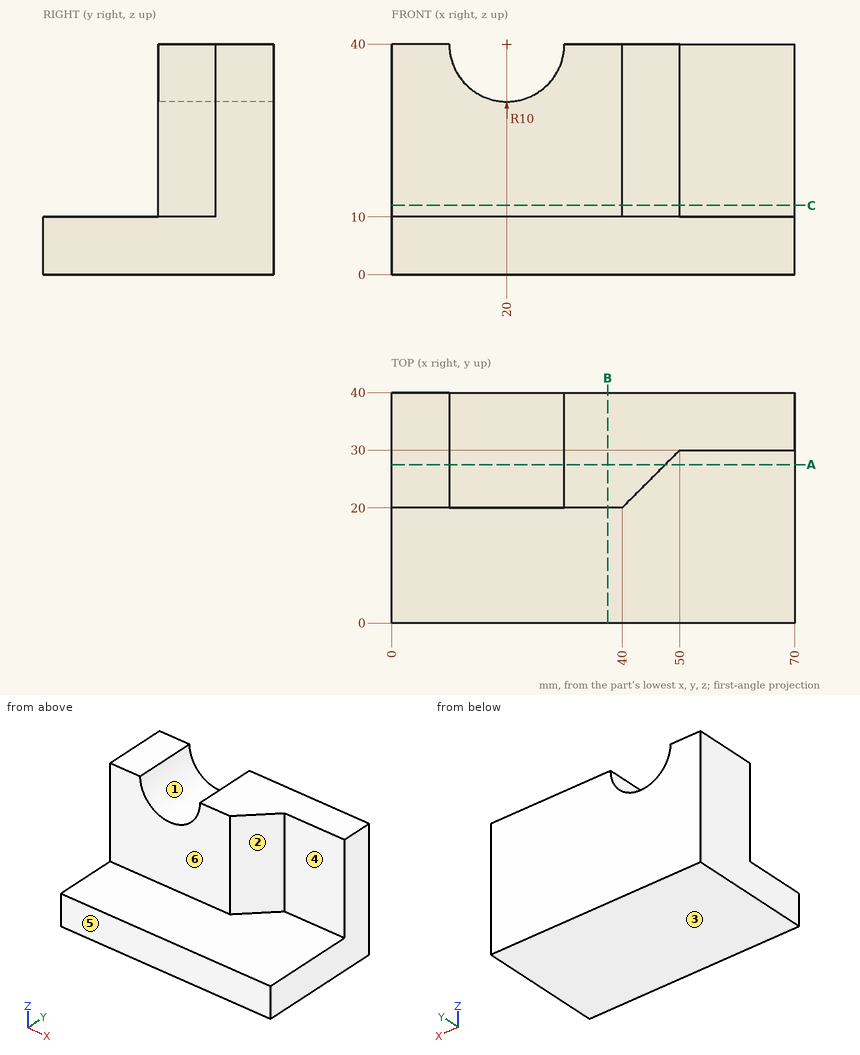
Could you check a few things on this drawing? It's one solid part, dimensions in mm from its lowest x, y, z. A direction names the side the tool comes from. Round coordinates to 2 decimals unless told otherwise and drop trailing zeros. Loops run counter-clockwise (first coordinate to the right, second up) from the corner with the lowest first, then second, coordinate; pieces in that order, holes last. Notation, with made-up numbers: (-7, 88.5) -> (43, 88.5) arc R14 ccw to (43, 114.5) -> close; hole circle Ø4 at (64.25, 4.5). An arc over 180 degrees is marked (long way). One line per item, written item: value. Start each with the question number.
1. For the marked faces 4, 5 and 6, which set-ups out of +Z, -Z, +X, -X, +Y, -Y let a thin tool reach every point of the face, with its end or its side?
2. If we section it at B-B, the plane x = 37.5: Write out the boundary of the cut face in (y, z).
3. If we section it at C-C, the plane z = 12: Write out the boundary of the cut face in (x, y), then the cut area to 3 significant figures.
4. For pin 1 (22 mm diameter, centred on x = 62.5, z = 32, fed in from -Y); pin 2 (2 mm diameter, centred on x = 53, y = 13.5, fed in from +Z); pin 3 (1 mm diameter, centred on y = 26, z = 33.5, fed in from +X), each with a flat end and sliding along its axis, tell me the tip position at first contact or that it passes through.
5. If we section it at A-A, the plane y = 27.5: Write out the boundary of the cut face in (x, z), then the cut area to 3 significant figures.
6. If we mould it in two halves opening along X, with no side actions, what happens to the marked faces 1, 2 and 3? For each: pulls with the +X half, pulls with the -X half, needs draft (parallel to the pull), parting line crosses it, or undercut.
7. If I drill on probe 1 along Y at (x, z) = (62.5, 15.5); probe 2 along Z at (x, y) = (21, 2); probe 3 along Y at (x, z) = (13, 16), over which ranges is the centre line in solid material (lowest first)?
Calculated:
1. face 4: +Z, +X, -Y
1. face 5: +Z, -Z, +X, -X, -Y
1. face 6: +Z, +X, -X, -Y
2. outline: (0, 0) -> (40, 0) -> (40, 40) -> (20, 40) -> (20, 10) -> (0, 10) -> close
3. outline: (0, 20) -> (40, 20) -> (50, 30) -> (70, 30) -> (70, 40) -> (0, 40) -> close
3. area: 1,150 mm²
4. pin 1: stops at y = 30
4. pin 2: stops at z = 10
4. pin 3: stops at x = 46.5
5. outline: (0, 0) -> (70, 0) -> (70, 10) -> (47.5, 10) -> (47.5, 40) -> (30, 40) arc R10 cw to (10, 40) -> (0, 40) -> close
5. area: 1,970 mm²
6. face 1: undercut
6. face 2: pulls with the +X half
6. face 3: needs draft
7. probe 1: y = 30 to 40
7. probe 2: z = 0 to 10
7. probe 3: y = 20 to 40
